Read the model definition and answer for the solid it produces. Units are mm, in the model's axes. A direction names the side the tool comes from. Coordinates: 2 decimals unless noted, no trailing zeros. Write each loop counter-clockwise with the first axis right and the second up, starting at its lowest first coordinate (ties: lowest second). Pieces come first, ordered by that corner, then holes. Notation, with made-up numbers: (-5.75, 44.25) -> (5.25, 44.25) arc R18 ccw to (5.25, 67.25) -> close; hole circle Ø5 at (15, 63.25). An arc over 180 degrees is marked (long way). Use CSV: the item, a comma, the result in double quotes. Start each with the question number.
from build123d import *

# Parameters (mm, degrees)
SKETCH1_R           = 5
SKETCH1_R_2         = 4.75
BOSS_EXTRUDE1_DEPTH = 3
BOSS_EXTRUDE2_START = -0.5
SKETCH2_R           = 5
SKETCH2_R_2         = 0.75
BOSS_EXTRUDE2_DEPTH = 0.5
SKETCH3_R           = 0.75
SKETCH3_R_2         = 1.25
BOSS_EXTRUDE3_DEPTH = 1
SKETCH4_R           = 0.25
CUT_EXTRUDE1_DEPTH  = 0.5
SKETCH5_W           = 2.8
SKETCH5_H           = 4.5
CUT_EXTRUDE2_DEPTH  = 0.5
SKETCH6_R           = 0.4
CUT_EXTRUDE3_DEPTH  = 0.5
SKETCH7_R           = 0.4
CUT_EXTRUDE4_DEPTH  = 0.2


with BuildPart() as part:
    # Sketch1 → Boss-Extrude1 (new body)
    with BuildSketch(Plane(origin=(0, 0, 0), x_dir=(1, 0, 0), z_dir=(0, 1, 0))):
        with Locations(Location((0, 0, 0), (0, 0, 270))):
            Circle(SKETCH1_R)
        with Locations(Location((0, 0, 0), (0, 0, 270))):
            Circle(SKETCH1_R_2, mode=Mode.SUBTRACT)
    extrude(amount=BOSS_EXTRUDE1_DEPTH)

    # Sketch2 → Boss-Extrude2 (add)
    with BuildSketch(Plane(origin=(0, 3, 0), x_dir=(1, 0, 0), z_dir=(0, 1, 0)).offset(BOSS_EXTRUDE2_START)):
        with Locations(Location((0, 0, 0), (0, 0, 270))):
            Circle(SKETCH2_R)
        with Locations(Location((0, 0, 0), (0, 0, 270))):
            Circle(SKETCH2_R_2, mode=Mode.SUBTRACT)
    extrude(amount=BOSS_EXTRUDE2_DEPTH)

    # Sketch3 → Boss-Extrude3 (add)
    with BuildSketch(Plane(origin=(0, 3, 0), x_dir=(1, 0, 0), z_dir=(0, 1, 0))):
        with BuildLine():
            Line((-4.898979486, -1), (4.898979486, -1))
            ThreePointArc((4.898979486, -1), (4.795459086, 1.415475947), (3.570714214, 3.5))
            Line((3.570714214, 3.5), (-3.570714214, 3.5))
            ThreePointArc((-3.570714214, 3.5), (-4.795459086, 1.415475947), (-4.898979486, -1))
        make_face()
        with Locations(Location((0, 0, 0), (0, 0, 270))):
            Circle(SKETCH3_R, mode=Mode.SUBTRACT)
        with Locations(Location((3, 2, 0), (0, 0, 270))):
            Circle(SKETCH3_R_2, mode=Mode.SUBTRACT)
        with Locations(Location((-3, 2, 0), (0, 0, 270))):
            Circle(SKETCH3_R_2, mode=Mode.SUBTRACT)
    extrude(amount=BOSS_EXTRUDE3_DEPTH)

    # Sketch4 → Cut-Extrude1 (cut)
    with BuildSketch(Plane(origin=(0, 3, 0), x_dir=(1, 0, 0), z_dir=(0, 1, 0))):
        with Locations(Location((-3, 2, 0), (0, 0, 270))):
            Circle(SKETCH4_R)
        with Locations(Location((3, 2, 0), (0, 0, 270))):
            Circle(SKETCH4_R)
    extrude(amount=-CUT_EXTRUDE1_DEPTH, mode=Mode.SUBTRACT)

    # Sketch5 → Cut-Extrude2 (cut)
    with BuildSketch(Plane(origin=(0, 4, 0), x_dir=(1, 0, 0), z_dir=(0, 1, 0))):
        with Locations((0, 1.25)):
            Rectangle(SKETCH5_W, SKETCH5_H)
    extrude(amount=-CUT_EXTRUDE2_DEPTH, mode=Mode.SUBTRACT)

    # Sketch6 → Cut-Extrude3 (cut)
    with BuildSketch(Plane(origin=(0, 3, 0), x_dir=(1, 0, 0), z_dir=(0, 1, 0))):
        with Locations(Location((0, -3.75, 0), (0, 0, 270))):
            Circle(SKETCH6_R)
        with Locations(Location((2.410453536, -2.872666662, 0), (0, 0, 270))):
            Circle(SKETCH6_R)
        with Locations(Location((-2.410453536, -2.872666662, 0), (0, 0, 270))):
            Circle(SKETCH6_R)
    extrude(amount=-CUT_EXTRUDE3_DEPTH, mode=Mode.SUBTRACT)

    # Sketch7 → Cut-Extrude4 (cut)
    # profile 1 of 3: a face of its own
    with BuildSketch(Plane(origin=(0, 3, 0), x_dir=(1, 0, 0), z_dir=(0, 1, 0))):
        with BuildLine():
            Line((-0.75, -3.75), (-0.75, -5.45))
            Line((-0.75, -5.45), (0.75, -5.45))
            Line((0.75, -5.45), (0.75, -3.75))
            ThreePointArc((0.75, -3.75), (0, -3), (-0.75, -3.75))
        make_face()
        with Locations(Location((0, -3.75, 0), (0, 0, 270))):
            Circle(SKETCH7_R, mode=Mode.SUBTRACT)
    # profile 2 of 3: a face of its own
    with BuildSketch(Plane(origin=(0, 3, 0), x_dir=(1, 0, 0), z_dir=(0, 1, 0))):
        with BuildLine():
            Line((-2.92865914, -4.657032922), (-1.835920204, -3.354757369))
            ThreePointArc((-1.835920204, -3.354757369), (-1.928362829, -2.298133329), (-2.984986869, -2.390575954))
            Line((-2.984986869, -2.390575954), (-4.077725805, -3.692851508))
            Line((-4.077725805, -3.692851508), (-2.92865914, -4.657032922))
        make_face()
        with Locations(Location((-2.410453536, -2.872666662, 0), (0, 0, 270))):
            Circle(SKETCH7_R, mode=Mode.SUBTRACT)
    # profile 3 of 3: a face of its own
    with BuildSketch(Plane(origin=(0, 3, 0), x_dir=(1, 0, 0), z_dir=(0, 1, 0))):
        with BuildLine():
            Line((2.984986869, -2.390575954), (4.077725805, -3.692851508))
            Line((4.077725805, -3.692851508), (2.92865914, -4.657032922))
            Line((2.92865914, -4.657032922), (1.835920204, -3.354757369))
            ThreePointArc((1.835920204, -3.354757369), (1.928362829, -2.298133329), (2.984986869, -2.390575954))
        make_face()
        with Locations(Location((2.410453536, -2.872666662, 0), (0, 0, 270))):
            Circle(SKETCH7_R, mode=Mode.SUBTRACT)
    extrude(amount=-CUT_EXTRUDE4_DEPTH, mode=Mode.SUBTRACT)


solid = part.part
1) Find the intervals of material crossed by line 1 along X through (y, z) = (3.3, 0); line 2 along X through (y, z) = (3.4, -2); line 3 along X through (y, z) = (2.9, -2), in increasing order.
2) Section A-A, the plane y = 3.7 is taken. Give the vertices of the cut face in (x, z), plus the area to 3 significant figures.
3) Section C-C, the plane x = 0 is taken. Give the vertices of the cut face in (y, z).
4) Section B-B, the plane z = 0 is taken. Give the vertices of the cut face in (x, y).
5) Which of the six approach directions +Z, -Z, +X, -X, +Y, -Y give full straight-line access (tool end or side, diameter ignored) to faces 4 (the face through (0, 3.5, -1)), 5 (the face through (0, 3.3, -3.5)), 6 (the face through (0, 2.8, 4.4)), 7 (the face through (-3.3, 3, -1.7)), 8 (the face through (-2.89, 1.23, -3.77))?
6) Section D-D, the plane z = -3 is taken. Give the vertices of the cut face in (x, y), plus the area to 3 significant figures.
7) The mould has two halves that part along Z. Classify faces 1 (the face through (3, 4, 0)), 2 (the face through (3.38, 3.49, -0.81)), 3 (the face through (-0.1, 3.3, 1)): pulls with the +Z half, pulls with the -Z half, needs draft (parallel to the pull), parting line crosses it, or undercut.
8) Each of these flat-tipped pins is pushed along its axis until it touches: pin 1 (1.5 mm diameter, centred on x = 3, z = -2, fed in from +Y); pin 2 (1 mm diameter, centred on x = 4, y = 2.5, fed in from -Z); pin 3 (1.5 mm diameter, centred on y = 3, z = -3.5, fed in from -X); pin 4 (3 mm diameter, centred on x = -3, z = -2, fed in from +Y). Where does it stop, or does it pass through?
The answers:
1,line 1,"x = -5 to -0.75, 0.75 to 5"
1,line 2,"x = -4.58 to -4.25, -1.75 to 1.75, 4.25 to 4.58"
1,line 3,"x = -4.58 to -3.25, -2.75 to 2.75, 3.25 to 4.58"
2,outline,"(-4.9, 1) arc R5 ccw to (-3.57, -3.5) -> (-1.4, -3.5) -> (-1.4, 1) -> close; (1.4, -3.5) -> (3.57, -3.5) arc R5 ccw to (4.9, 1) -> (1.4, 1) -> close; hole circle Ø2.5 at (-3, -2); hole circle Ø2.5 at (3, -2)"
2,area,"19.4 mm^2"
3,outline,"(0, -5) -> (3, -5) -> (3, -3.5) -> (3.5, -3.5) -> (3.5, -0.75) -> (2.5, -0.75) -> (2.5, -4.75) -> (0, -4.75) -> close; (0, 4.75) -> (2.5, 4.75) -> (2.5, 4.15) -> (2.8, 4.15) -> (2.8, 5) -> (0, 5) -> close; (2.5, 0.75) -> (3.5, 0.75) -> (3.5, 1) -> (3, 1) -> (3, 3) -> (2.8, 3) -> (2.8, 3.35) -> (2.5, 3.35) -> close"
4,outline,"(-5, 0) -> (-4.75, 0) -> (-4.75, 2.5) -> (-0.75, 2.5) -> (-0.75, 3.5) -> (-1.4, 3.5) -> (-1.4, 4) -> (-5, 4) -> close; (0.75, 2.5) -> (4.75, 2.5) -> (4.75, 0) -> (5, 0) -> (5, 4) -> (1.4, 4) -> (1.4, 3.5) -> (0.75, 3.5) -> close"
5,face 4,"+Z, -Z, +Y"
5,face 5,"-Z, +X, -X, +Y"
5,face 6,"+Z, +Y"
5,face 7,"+Y"
5,face 8,"-Y"
6,outline,"(-4, 0) -> (-3.68, 0) -> (-3.68, 2.5) -> (3.68, 2.5) -> (3.68, 0) -> (4, 0) -> (4, 4) -> (3.75, 4) -> (3.75, 3) -> (2.25, 3) -> (2.25, 4) -> (1.4, 4) -> (1.4, 3.5) -> (-1.4, 3.5) -> (-1.4, 4) -> (-2.25, 4) -> (-2.25, 3) -> (-3.75, 3) -> (-3.75, 4) -> (-4, 4) -> close"
6,area,"9.19 mm^2"
7,face 1,"needs draft"
7,face 2,"undercut"
7,face 3,"pulls with the +Z half"
8,pin 1,"stops at y = 3"
8,pin 2,"stops at z = -3.57"
8,pin 3,"stops at x = -4.18"
8,pin 4,"stops at y = 4"
